from build123d import *

# Parameters (mm, degrees)
F1_DEPTH      = 3.81
F2_SIZE       = 5.08
F3_T1_DEPTH   = 45.7068968586
F3_T3_DEPTH   = 45.7068968586
F5_DEPTH      = 25.4
F5_DEPTH_BACK = 3.81


# Not quite as in the source:
# - a fillet or chamfer that OpenCascade refuses, or shapes differently, is made with other operations: its cross-section is extruded or revolved along the edge and cut away or added


with BuildPart() as f1:
    # F0 (on Top) → F1 (new body)
    with BuildSketch(Plane.XY):
        Polygon((-0.2622354642, -15.1205231096), (13.2258748636, 7.3331589811), (-12.9636393994, 7.7873641286), align=None)
    extrude(amount=F1_DEPTH)

    # F2
    f2_edges = [f1.edges().sort_by_distance(p)[0] for p in [
        (-0.262235, -15.120523, 1.905),
    ]]
    chamfer(f2_edges, length=F2_SIZE)

    # F3: fillet of radius 5.08 on 2 edges, made by hand

    # F3_s2 → F3_t1 (cut)
    with BuildSketch(Plane(origin=(-10.4602488885, -17.4131955793, 0), x_dir=(0, 0, 1), z_dir=(0.5149420555, 0.8572249877, 0))):
        with BuildLine():
            ThreePointArc((0, 7.5613984578), (2.7460926284, 5.7535615814), (3.81, 2.6427096081))
            Line((3.81, 2.6427096081), (3.81, 7.5613984578))
            Line((3.81, 7.5613984578), (0, 7.5613984578))
        make_face()
    extrude(amount=F3_T1_DEPTH, mode=Mode.SUBTRACT)

    # F3_s4 → F3_t3 (cut)
    with BuildSketch(Plane(origin=(-12.3134758372, 22.2082312655, 0), x_dir=(0, 0, 1), z_dir=(0.4849075883, -0.8745653954, 0))):
        with BuildLine():
            ThreePointArc((3.81, 2.6427096081), (2.7460926284, 5.7535615814), (0, 7.5613984578))
            Line((0, 7.5613984578), (3.81, 7.5613984578))
            Line((3.81, 7.5613984578), (3.81, 2.6427096081))
        make_face()
    extrude(amount=F3_T3_DEPTH, mode=Mode.SUBTRACT)

    # F4 (on face) → F5 (join, two sides)
    with BuildSketch(Plane.XY.offset(3.81)) as f5_sk:
        Polygon((1.27, 7.5405099022), (1.27, 8.8325355317), (-1.27, 8.8325355317), (-1.27, 7.5845611611), align=None)
    extrude(amount=F5_DEPTH)
    extrude(f5_sk.sketch, amount=-F5_DEPTH_BACK)


solid = f1.part
Could you check a few things on this model? Use its own coordinates, in mm. Give positions to 0.01 mm unless a question says otherwise; leave off trailing zeros. Write each loop counter-clockwise with the first axis right and the second up, starting at its lowest first coordinate (ties: lowest second). Pieces come first, ordered by that corner, then holes. Notation, with made-up numbers: (71.25, -28.75) -> (80.25, -28.75) arc R19 ccw to (80.25, -6.75) -> close; hole circle Ø6 at (53.5, 25). An arc over 180 degrees is marked (long way). Answer as CSV lines item,"result". Start each with the question number.
(1) I'm going to push flat-ended pins straight in: pin 1 Ø10.5 at (x, y) = (2, -1.5) entering from +Z; pin 2 Ø1 at (y, z) = (8.5, 12) entering from -X; pin 3 Ø12 at (x, z) = (4, 6.5) entering from -Y. Where does each tip first touch, or does it pass through?
(2) If we section it at A-A, the plane z = 15.25: Write out the boundary of the cut face in (x, y).
(3) Please list where these lines run through material, in increasing order: line 1 (Y direction, x = 1, z = 16.5); line 2 (Z direction, x = -4.5, y = 4.5); line 3 (Y direction, x = -0.5, z = 16).
Answer list:
1,pin 1,"z = 3.81"
1,pin 2,"x = -1.27"
1,pin 3,"y = -10.76"
2,outline,"(-1.27, 7.58) -> (1.27, 7.54) -> (1.27, 8.83) -> (-1.27, 8.83) -> close"
3,line 1,"7.55 to 8.83"
3,line 2,"0 to 3.81"
3,line 3,"7.57 to 8.83"
